The listing builds one solid part. Answer for the finished solid, in the listing's coordinates (mm). A direction names the side the tool comes from. Give positions to 0.01 mm unless a question says otherwise; leave off trailing zeros. Write each loop counter-clockwise with the first axis right and the second up, starting at its lowest first coordinate (ties: lowest second). Pieces come first, ordered by that corner, then holes. Notation, with made-up numbers: M -35,-36 L -18,-36 A31 cw -18,0 Z; hole C 35,64 d8. An arc over 180 degrees is marked long. Answer as a JSON object with one key per item and string values.
```python
from build123d import *

# Parameters (mm, degrees)
F0_W     = 15.0114
F0_H     = 17.4625
F0_W_2   = 7.2136
F0_H_2   = 10.287
F2_R     = 1.5875
F3_SIZE  = 0.79375
F4_SIZE2 = 6.35
F4_SIZE  = 0.6604


with BuildPart() as f1:
    # F0 (on Right) → F1 (revolve)
    with BuildSketch(Plane.YZ):
        with Locations((14.7193, 16.66875)):
            Rectangle(F0_W, F0_H)
        with Locations((3.6068, 30.5435)):
            Rectangle(F0_W_2, F0_H_2)
        with Locations((3.6068, 16.66875)):
            Rectangle(F0_W_2, F0_H)
    revolve(axis=Axis((0, 11.1125, 0), (0, 1, 0)))

    # F2
    f2_edges = [f1.edges().sort_by_distance(p)[0] for p in [
        (0, 7.2136, -25.4),
    ]]
    fillet(f2_edges, radius=F2_R)

    # F3
    f3_edges = [f1.edges().sort_by_distance(p)[0] for p in [
        (0, 22.225, -25.4),
    ]]
    chamfer(f3_edges, length=F3_SIZE)

    # F4
    f4_edges = [f1.edges().sort_by_distance(p)[0] for p in [
        (0, 0, -35.687),
        (0, 7.2136, -35.687),
    ]]
    f4_side = f1.faces().sort_by_distance((0, 3.6068, -35.687))[0]
    chamfer(f4_edges, length=F4_SIZE, length2=F4_SIZE2, reference=f4_side)


solid = f1.part
```
1. A cutting plane is placed at B-B, the plane x = 0. Give the vertices of the cut face in (y, z) (1 decimal).
Verdict:
{"outline": "M 0,-29.3 L 0.7,-35.7 L 6.6,-35.7 L 7.2,-29.3 L 7.2,-27 A1.6 cw 8.8,-25.4 L 21.4,-25.4 L 22.2,-24.6 L 22.2,-7.9 L 0,-7.9 Z; M 0,7.9 L 22.2,7.9 L 22.2,24.6 L 21.4,25.4 L 8.8,25.4 A1.6 cw 7.2,27 L 7.2,29.3 L 6.6,35.7 L 0.7,35.7 L 0,29.3 Z"}
2. Consider line 1 along X through (y, z) = (16.25, 0); line 2 along Y through (x, z) = (17.5, -22.5); line 3 along Z through (x, y) = (3, 20.5). Determine where each line is inside the solid, lowest interval first.
Verdict:
{"line 1": "x = -25.4 to -7.94, 7.94 to 25.4", "line 2": "y = 0 to 7.21", "line 3": "z = -25.22 to -7.35, 7.35 to 25.22"}
3. The mould has two halves that part along X. Classify faces 3 (the flat face through (6, 22.225, 6)), 4 (the cylindrical face through (30.09, 3.65, 19.19)), 5 (the cylindrical face through (-7.75, 11.27, -1.72)): released by +X, released by -X, zero draft, split by the parting line, or undercut.
Verdict:
{"face 3": "zero draft", "face 4": "split by the parting line", "face 5": "undercut"}
4. For faces 1 (the cylindrical face through (-24.796, 15.205, -5.506)), 2 (the flat face through (-6, 0, 6)), determine the directions among +Z, -Z, +X, -X, +Y, -Y from which every point of the face is accessible in a straight line to the end or side of a thin tool.
Verdict:
{"face 1": "+Y", "face 2": "+Z, -Z, +X, -X, -Y"}
5. A cutting plane is placed at D-D, the plane y = 12.5. Give the vertices of the cut face in (x, z) (1 decimal), plus the area to 3 significant figures.
Verdict:
{"outline": "C 0,0 d50.8; hole C 0,0 d15.9", "area": "1,830 mm2"}
6. A cutting plane is placed at A-A, the plane z = 0. Give the vertices of the cut face in (x, y) (1 decimal), plus the area to 3 significant figures.
Verdict:
{"outline": "M -35.7,0.7 L -29.3,0 L -7.9,0 L -7.9,22.2 L -24.6,22.2 L -25.4,21.4 L -25.4,8.8 A1.6 cw -27,7.2 L -29.3,7.2 L -35.7,6.6 Z; M 7.9,0 L 29.3,0 L 35.7,0.7 L 35.7,6.6 L 29.3,7.2 L 27,7.2 A1.6 cw 25.4,8.8 L 25.4,21.4 L 24.6,22.2 L 7.9,22.2 Z", "area": "917 mm2"}
7. A cutting plane is placed at C-C, the plane y = 4.5. Give the vertices of the cut face in (x, z) (1 decimal), plus the area to 3 significant figures.
Verdict:
{"outline": "C 0,0 d71.4; hole C 0,0 d15.9", "area": "3,800 mm2"}
8. Flat-ended cylindrical pins translate along their axes: pin 1 (12 mm diameter, centred on y = 16.5, z = -22.5, fed in from +X); pin 2 (1.5 mm diameter, centred on x = -24.5, z = -27.5, fed in from -Y); pin 3 (1.5 mm diameter, centred on y = 15, z = 15, fed in from +X); pin 4 (5 mm diameter, centred on x = -28, z = 17, fed in from +Y). Find the tip coordinate at first contact, or state that the pin passes through.
Verdict:
{"pin 1": "stops at x = 19.31", "pin 2": "passes through", "pin 3": "stops at x = 21.03", "pin 4": "stops at y = 7.12"}
